Model file for the job. Use its own axes, mm. A direction names the side the tool comes from. Give positions to 0.01 mm unless a question says otherwise; leave off trailing zeros. Order: outer loops, then holes, each group sorted by start corner. A loop starts at its lowest first (then second) coordinate and runs counter-clockwise, first axis right, second up. Notation, with made-up numbers: (41, 58) - (65, 58) arc R34 ccw to (65, 89) - close; hole circle Ø1 at (5.25, 28). An arc over 180 degrees is marked (long way). Use CSV: the item, a comma, the result in double quotes. Start each with the question number.
(1) Tool access for faces 5 (the flat face through (-67.5, -48, -1)), 6 (the flat face through (75, -44, 1)), 7 (the flat face through (-12.5, -77, 71)): list every direction of +Z, -Z, +X, -X, +Y, -Y with a clear straight run to the whole face (end or side of a thin tool).
(2) Band-saw the part on A-A, the plane z = -32.5. Give the cut face in (x, y).
(3) Drop flat-ended pins along their axis: pin 1 Ø3.5 at (x, z) = (53.95, 0) entering from +Y; pin 2 Ø3 at (x, z) = (28, 53) entering from -Y; pin 3 Ø4 at (x, z) = (-23.5, 71.5) entering from -Y. Give the stop position or say it passes through.
(4) Probe L1, parallel to X at y = -2.45, z = 53.95; L2, parallel to X at y = -40, z = -41.5. List the from-to ranges inside material, lowest first.
(5) Band-saw the part on C-C, the plane y = -39. Give the cut face in (x, z), then the cut area to 4 significant figures.
(6) Band-saw the part on B-B, the plane x = 0. Give the cut face in (y, z), then the cut area to 3 significant figures.
(7) Band-saw the part on D-D, the plane x = 53.95. Give the cut face in (y, z), then the cut area to 3 significant figures.
(8) Pull direction Z, two halves, no side cores. Call faces 1 (the flat face through (1, -44, 75)), 2 (the flat face through (68, 0, -1)), 3 (the flat face through (-1, -48, -67.5)), 4 (the cylindrical face through (-54.796, 2.465, 28.501)): +Z half, -Z half, draft (parallel to the pull), parting line (faces both ways), or undercut.
from build123d import *
from build123d.topology import SkipClean

# Parameters (mm, degrees)
SKETCH1_R           = 61.765082955
SKETCH1_R_2         = 47.5
BOSS_EXTRUDE1_DEPTH = 5
SKETCH7_R           = 2.25
CUT_EXTRUDE1_DEPTH  = 9.5
SKETCH9_W           = 150
SKETCH9_H           = 150
SKETCH9_R           = 2.25
SKETCH9_R_2         = 47.5
BOSS_EXTRUDE2_DEPTH = 90
CUT_EXTRUDE2_DEPTH  = 60
SKETCH10_W          = 135
SKETCH10_H          = 135
CUT_EXTRUDE4_DEPTH  = 85


with BuildPart() as part:
    # Sketch1 → Boss-Extrude1 (new body)
    with BuildSketch(Plane(origin=(0, 0, 0), x_dir=(1, 0, 0), z_dir=(0, 1, 0))):
        with Locations(Location((0, 0, 0), (0, 0, 270))):
            Circle(SKETCH1_R)
        with Locations(Location((0, 0, 0), (0, 0, 270))):
            Circle(SKETCH1_R_2, mode=Mode.SUBTRACT)
    extrude(amount=BOSS_EXTRUDE1_DEPTH)

    # Sketch7 → Cut-Extrude1 (cut)
    with BuildSketch(Plane(origin=(0, 5, 0), x_dir=(1, 0, 0), z_dir=(0, 1, 0))):
        with Locations(Location((0, 53.95, 0), (0, 0, 270))):
            Circle(SKETCH7_R)
        with Locations(Location((0, -53.95, 0), (0, 0, 270))):
            Circle(SKETCH7_R)
        with Locations(Location((53.95, 0, 0), (0, 0, 270))):
            Circle(SKETCH7_R)
        with Locations(Location((-53.95, 0, 0), (0, 0, 270))):
            Circle(SKETCH7_R)
    extrude(amount=-CUT_EXTRUDE1_DEPTH, mode=Mode.SUBTRACT)

    # Sketch9 → Boss-Extrude2 (add)
    with SkipClean():  # the faces are left unmerged after this step: merging them gives an invalid solid
        with BuildSketch(Plane(origin=(0, 0, 0), x_dir=(-1, 0, 0), z_dir=(0, -1, 0))):
            Rectangle(SKETCH9_W, SKETCH9_H)
            with Locations(Location((0, -53.95, 0), (0, 0, 90))):
                Circle(SKETCH9_R, mode=Mode.SUBTRACT)
            with Locations(Location((53.95, 0, 0), (0, 0, 90))):
                Circle(SKETCH9_R, mode=Mode.SUBTRACT)
            with Locations(Location((0, 53.95, 0), (0, 0, 270))):
                Circle(SKETCH9_R, mode=Mode.SUBTRACT)
            with Locations(Location((-53.95, 0, 0), (0, 0, 270))):
                Circle(SKETCH9_R, mode=Mode.SUBTRACT)
            with Locations(Location((0, 0, 0), (0, 0, 90))):
                Circle(SKETCH9_R_2, mode=Mode.SUBTRACT)
        extrude(amount=BOSS_EXTRUDE2_DEPTH)

    # 3DSketch2 → Cut-Extrude2 (cut)
    with SkipClean():  # the faces are left unmerged after this step: merging them gives an invalid solid
        with BuildSketch(Plane(origin=(-42.5, -65, 75), x_dir=(0.7071067811865476, -0.7071067811865476, 0), z_dir=(0, 0, 1))):
            Polygon((0, 0), (21.213203436, 21.213203436), (42.426406871, 0), (21.213203436, -21.213203436), align=None)
        extrude(amount=-CUT_EXTRUDE2_DEPTH, mode=Mode.SUBTRACT)

    # Sketch10 → Cut-Extrude4 (cut)
    with SkipClean():  # the faces are left unmerged after this step: merging them gives an invalid solid
        with BuildSketch(Plane.XZ.offset(90)):
            Rectangle(SKETCH10_W, SKETCH10_H)
        extrude(amount=-CUT_EXTRUDE4_DEPTH, mode=Mode.SUBTRACT)


solid = part.part
Answer block:
1,face 5,"-Y"
1,face 6,"+Z, -Z, +X, +Y, -Y"
1,face 7,"+Z, -Y"
2,outline,"(-75, -90) - (-67.5, -90) - (-67.5, -5) - (-34.64, -5) - (-34.64, 5) - (-52.52, 5) - (-52.52, 0) - (-75, 0) - close; (34.64, -5) - (67.5, -5) - (67.5, -90) - (75, -90) - (75, 0) - (52.52, 0) - (52.52, 5) - (34.64, 5) - close"
3,pin 1,"passes through"
3,pin 2,"stops at y = -5"
3,pin 3,"stops at y = -65"
4,L1,"x = -75 to -2.25, 2.25 to 75"
4,L2,"x = -75 to -67.5, 67.5 to 75"
5,outline,"(-75, -75) - (75, -75) - (75, 75) - (-75, 75) - close; hole (-67.5, -67.5) - (67.5, -67.5) - (67.5, 67.5) - (-67.5, 67.5) - close"
5,area,"4,275 mm2"
6,outline,"(-90, -75) - (0, -75) - (0, -61.77) - (5, -61.77) - (5, -56.2) - (-5, -56.2) - (-5, -67.5) - (-90, -67.5) - close; (-90, 67.5) - (-5, 67.5) - (-5, 56.2) - (5, 56.2) - (5, 61.77) - (0, 61.77) - (0, 75) - (-90, 75) - close; (-5, -51.7) - (5, -51.7) - (5, -47.5) - (-5, -47.5) - close; (-5, 47.5) - (5, 47.5) - (5, 51.7) - (-5, 51.7) - close"
6,area,"1,600 mm2"
7,outline,"(-90, -75) - (0, -75) - (0, -30.07) - (5, -30.07) - (5, -2.25) - (-5, -2.25) - (-5, -67.5) - (-90, -67.5) - close; (-90, 67.5) - (-5, 67.5) - (-5, 2.25) - (5, 2.25) - (5, 30.07) - (0, 30.07) - (0, 75) - (-90, 75) - close"
7,area,"2,280 mm2"
8,face 1,"+Z half"
8,face 2,"draft"
8,face 3,"undercut"
8,face 4,"parting line"
